Autodesk Inventor part; units mm, degrees
ref_plane "YZ Plane" through (0, 0, 0) normal (1, 0, 0) x (0, 1, 0)
ref_plane "XZ Plane" through (0, 0, 0) normal (0, 1, 0) x (-1, 0, 0)
ref_plane "XY Plane" through (0, 0, 0) normal (0, 0, 1) x (1, 0, 0)
sketch "スケッチ1" plane through (0, 0, 0) normal (0, 1, 0) x (-1, 0, 0)
  line L0 (4.5, 2.55) -> (-4.5, 2.55) construction
  line L1 (-4.5, 2.55) -> (-4.5, -2.55) construction
  line L2 (-4.5, -2.55) -> (4.5, -2.55) construction
  line L3 (4.5, -2.55) -> (4.5, 2.55) construction
  line L4 (4.5, 2.55) -> (-4.5, -2.55) construction
  line L5 (-4.5, 2.55) -> (4.5, -2.55) construction
  line L6 (5.4458, 0) -> (-6.2593, 0)
  line L7 (4.5, 0) -> (-4.5, 0)
  arc A0 (4.5, 0) -> (1.95, 2.55) centre (1.95, 0) ccw
  line L8 (-4.5, 2.55) -> (-4.5, 0)
  line L9 (1.95, 2.55) -> (-4.5, 2.55)
  point P0 (0, 0)
  dimension "d0" = 9
  dimension "d1" = 5.1
revolve "回転1" add sketch "スケッチ1" angle 360 about axis through (-5.4458, 0, 0) along (1, 0, 0)
sketch "スケッチ2" plane through (4.5, 0, 0) normal (1, 0, 0) x (0, 0, -1)
  line L0 (-3.2936, 0) -> (3.5532, 0)
  line L1 (0, -3.9082) -> (0, 3.9846)
  line L2 (-1.52, 0.25) -> (-1.02, 0.25)
  line L3 (-1.02, 0.25) -> (-1.02, -0.25)
  line L4 (-1.02, -0.25) -> (-1.52, -0.25)
  line L5 (-1.52, -0.25) -> (-1.52, 0.25)
  line L6 (-1.52, 0.25) -> (-1.02, -0.25) construction
  line L7 (-1.02, 0.25) -> (-1.52, -0.25) construction
  line L8 (1.52, 0.25) -> (1.02, 0.25)
  line L9 (1.02, 0.25) -> (1.02, -0.25)
  line L10 (1.02, -0.25) -> (1.52, -0.25)
  line L11 (1.52, 0.25) -> (1.02, -0.25) construction
  line L12 (1.02, 0.25) -> (1.52, -0.25) construction
  line L13 (1.52, -0.25) -> (1.52, 0.25)
  point P0 (0, 0)
  point P1 (-1.27, 0)
  point P2 (-1.27, 0)
  point P3 (1.27, 0)
  point P4 (1.27, 0)
  dimension "d9" = 0.5
  dimension "d10" = 0.5
  dimension "d11" = 1.27
extrude "押し出し1" add sketch "スケッチ2" along normal blind 2
sketch "スケッチ3" plane through (4.5, -0.25, 1.02) normal (0, -1, 0) x (1, 0, 0)
  line L0 (1.5, 0) -> (2, 0)
  line L1 (2, 0) -> (2, 0.5)
  line L2 (2, 0.5) -> (1.5, 0.5)
  line L3 (1.5, 0.5) -> (1.5, 0)
  line L4 (1.5, 0) -> (2, 0.5) construction
  line L5 (2, 0) -> (1.5, 0.5) construction
  line L6 (1.5, -2.04) -> (2, -2.04)
  line L7 (2, -2.04) -> (2, -2.54)
  line L8 (2, -2.54) -> (1.5, -2.54)
  line L9 (1.5, -2.54) -> (1.5, -2.04)
  line L10 (1.5, -2.04) -> (2, -2.54) construction
  line L11 (2, -2.04) -> (1.5, -2.54) construction
  point P0 (-4.5, -1.02)
  point P1 (1.75, 0.25)
  point P2 (1.75, -2.29)
  dimension "d14" = 0.5
  dimension "d15" = 0.5
  dimension "d16" = 0.5
  dimension "d17" = 0.5
extrude "押し出し2" add sketch "スケッチ3" along normal blind 4
properties part number "LED"
Build history of the part. All positions in model axes, mm. A direction names the side the tool comes from. Round coordinates to 2 decimals unless told otherwise and drop trailing zeros. Loops run counter-clockwise (first coordinate to the right, second up) from the corner with the lowest first, then second, coordinate; pieces in that order, holes last. Notation, with made-up numbers: (82.5, 7.25) -> (118.5, 7.25) arc R35 ccw to (118.5, 42.25) -> close; hole circle Ø11 at (70.5, 60.5). An arc over 180 degrees is marked (long way). One line per item, written item: value. Start each with the question number.
Q1. Drop flat-ended pins along their axis: pin 1 Ø0.6 at (y, z) = (-2.5, 1.5) entering from -X; pin 2 Ø0.6 at (y, z) = (-2, -1.5) entering from -X; pin 3 Ø0.6 at (x, z) = (5.5, 1) entering from +Y. Give the stop position or say it passes through.
Q2. Cut at C-C on z = 1.25. List the corners of the cut face in (x, y).
Q3. Cut at D-D on x = 1. List the corners of the cut face in (y, z).
Q4. Cut at B-B on y = 0. List the corners of the cut face in (x, z), plus the area to 3 significant figures.
Q5. Probe line 1 along Y through (x, z) = (1.75, -0.1); line 2 along X through (y, z) = (0.5, -1.75); line 3 along Y through (x, z) = (0.5, 1.55). List the from-to ranges inside material, lowest first.
Q6. 3-axis set-ups, long thin cutter, end or side, ignore diameter. For faces 1 (the face through (6.2, -1.5, 1.02)), 2 (the face through (6.2, -1.7, 1.52)): which of +Z, -Z, +X, -X, +Y, -Y reach the whole face in a straight line?
Q7. Cut at A-A on y = -3.25. List the corners of the cut face in (x, z).
Q8. Two-plate mould, pull along Z, no slides. Class faces 3 (the face through (6.2, -1.7, -1.52)), 4 (the face through (1.32, 2.26, 1.18)), 5 (the face through (6.2, -1.5, -1.02)): released by +Z, released by -Z, zero draft, split by the parting line, or undercut.
Computed:
1. pin 1: x = 6
1. pin 2: x = -3.24
1. pin 3: y = 0.25
2. outline: (-1.95, -2.22) -> (4.5, -2.22) -> (4.5, -0.25) -> (6, -0.25) -> (6, -4.25) -> (6.5, -4.25) -> (6.5, 0.25) -> (4.5, 0.25) -> (4.5, 2.22) -> (-1.95, 2.22) arc R2.22 ccw to start
3. outline: circle Ø5.1 at (0, 0)
4. outline: (-1.95, -2.55) -> (4.5, -2.55) -> (4.5, -1.52) -> (6.5, -1.52) -> (6.5, -1.02) -> (4.5, -1.02) -> (4.5, 1.02) -> (6.5, 1.02) -> (6.5, 1.52) -> (4.5, 1.52) -> (4.5, 2.55) -> (-1.95, 2.55) arc R2.55 ccw to start
4. area: 45.1 mm²
5. line 1: -2.55 to 2.55
5. line 2: -3.74 to 4.5
5. line 3: -2.02 to 2.02
6. face 1: +X, +Y, -Y
6. face 2: +Z, +X, +Y, -Y
7. outline: (6, -1.52) -> (6.5, -1.52) -> (6.5, -1.02) -> (6, -1.02) -> close; (6, 1.02) -> (6.5, 1.02) -> (6.5, 1.52) -> (6, 1.52) -> close
8. face 3: released by -Z
8. face 4: split by the parting line
8. face 5: undercut
